from build123d import *

# Parameters (mm, degrees)
SKETCH1_W          = 2
SKETCH1_H          = 36
CUT_EXTRUDE1_DEPTH = 6
FILLET1_R          = 1


with BuildPart() as part:
    # BodySke → BaseBody (revolve)
    with BuildSketch(Plane.XY, mode=Mode.PRIVATE) as basebody_sk:
        with BuildLine():
            Line((0, 0), (0, 16))
            Line((0, 16), (2, 18))
            Line((2, 18), (6, 18))
            Line((6, 18), (6, 12))
            Line((6, 12), (52, 12))
            Line((52, 12), (52, 10.088985))
            ThreePointArc((52, 10.088985), (52.322621881, 9.310106881), (53.1015, 8.987485))
            Line((53.1015, 8.987485), (54.4233, 8.987485))
            Line((54.4233, 8.987485), (55.435815, 10))
            Line((55.435815, 10), (79.8985, 10))
            Line((79.8985, 10), (81, 8.8985))
            Line((81, 8.8985), (81, 0))
            Line((81, 0), (0, 0))
        make_face()
    revolve(basebody_sk.sketch.rotate(Axis((-6.35, 0, 0), (1, 0, 0)), 90), axis=Axis((-6.35, 0, 0), (1, 0, 0)))

    # Sketch1 → Cut-Extrude1 (cut)
    with BuildSketch(Plane.ZY):
        with Locations((-17, 0)):
            Rectangle(SKETCH1_W, SKETCH1_H)
        with Locations((17, 0)):
            Rectangle(SKETCH1_W, SKETCH1_H)
    extrude(amount=-CUT_EXTRUDE1_DEPTH, mode=Mode.SUBTRACT)

    # Fillet1
    fillet1_edges = [part.edges().sort_by_distance(p)[0] for p in [
        (6, 0, -12),
    ]]
    fillet(fillet1_edges, radius=FILLET1_R)


solid = part.part
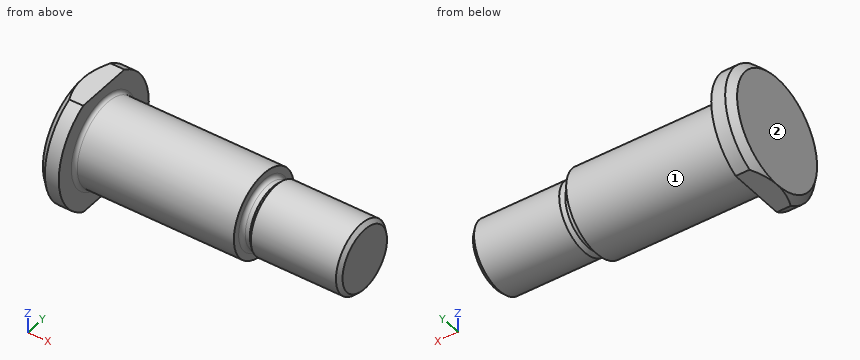
For this review, take the finished solid that the model builds, in its own axes (mm). Face numbers are marked on the shaded views. A direction names the side the tool comes from. Give positions to 0.01 mm unless a question says otherwise; leave off trailing zeros. Loops run counter-clockwise (first coordinate to the right, second up) from the corner with the lowest first, then second, coordinate; pieces in that order, holes last. Notation, with made-up numbers: M -1,22 L 6,22 A15 ccw 6,30 Z; hole C -7.5,40.25 d10. An arc over 180 degrees is marked long. Put each result on its own line as item: value. Start each with the question number.
(1) For pin 1 (3 mm diameter, centred on y = 9.5, z = -4.5, fed in from +X); pin 2 (10 mm diameter, centred on x = 55, y = 4, fed in from +Z); pin 3 (4 mm diameter, centred on x = 18, z = 1, fed in from -Y), all flat-tipped, find the tip position at first contact; note any pin that passes through.
(2) Wall thickness on L1, parallel to X at y = -11, z = -3.5; L2, parallel to Y at x = 28, z = -0.5; L3, parallel to X at y = 11.5, z = 9.5: over which ranges is each line inside the solid? List them lowest first.
(3) Add section A-A, the plane z = 0. Write out the cut boundary in (x, y), then the cut area to 3 significant figures.
(4) Machinability: for the marked faces 1 and 2, which of the approach directions +Z, -Z, +X, -X, +Y, -Y give a long, thin tool a straight path to every point of the face, cutting with its end or side? Answer none if there is none.
(5) Add section B-B, the plane x = 5. Write out the cut boundary in (y, z).
(6) Add section C-C, the plane x = 59.5. Write out the cut boundary in (y, z).
Result:
1. pin 1: stops at x = 80.89
1. pin 2: stops at z = 12
1. pin 3: stops at y = -12
2. L1: x = 0 to 52
2. L2: y = -11.99 to 11.99
2. L3: x = 0 to 6
3. outline: M 0,-16 L 2,-18 L 6,-18 L 6,-13 A1 cw 7,-12 L 52,-12 L 52,-10.09 A1.1 cw 53.1,-8.99 L 54.42,-8.99 L 55.44,-10 L 79.9,-10 L 81,-8.9 L 81,8.9 L 79.9,10 L 55.44,10 L 54.42,8.99 L 53.1,8.99 A1.1 cw 52,10.09 L 52,12 L 7,12 A1 cw 6,13 L 6,18 L 2,18 L 0,16 Z
3. area: 1,890 mm^2
4. face 1: +X
4. face 2: +Z, -Z, -X, +Y, -Y
5. outline: M -8.25,-16 L 8.25,-16 A18 ccw 8.25,16 L -8.25,16 A18 ccw Z
6. outline: C 0,0 d20
